Can you work these out from the drawing? Everything is in mm from the part's minimum corner. Round coordinates to 2 decimals unless told otherwise and drop trailing zeros. Write each loop counter-clockwise with the first axis right and the second up, starting at its lowest first coordinate (ties: lowest second). Pieces come first, ordered by that corner, then holes. Notation, with made-up numbers: (-30.75, 8.25) -> (22.25, 8.25) arc R8 ccw to (22.25, 14.25) -> close; hole circle Ø7 at (11, -21). An arc over 180 degrees is marked (long way). Write item = value, one per line. Start each with the question number.
1) Imagine slicing it at B-B, the plane z = 2.5. Please give me the cut outline in (x, y).
2) If I drill on line 1 (Y direction, x = 0.45, z = 5.25), over which ranges is the centre line in solid material (lowest first)?
3) Imagine slicing it at A-A, the plane x = 0.25. Please give me the cut outline in (y, z).
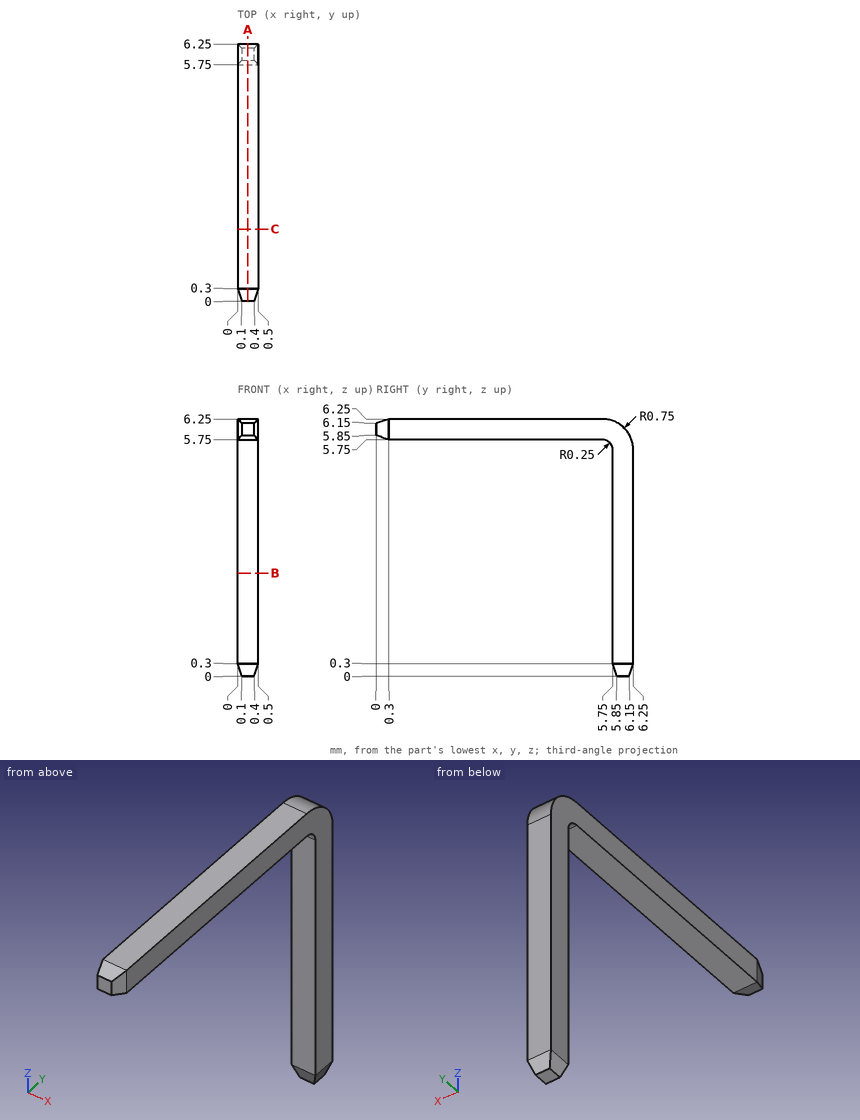
Reported:
q1.outline = (0, 5.75) -> (0.5, 5.75) -> (0.5, 6.25) -> (0, 6.25) -> close
q2.line_1 = 5.75 to 6.25
q3.outline = (0, 5.85) -> (0.3, 5.75) -> (5.5, 5.75) arc R0.25 cw to (5.75, 5.5) -> (5.75, 0.3) -> (5.85, 0) -> (6.15, 0) -> (6.25, 0.3) -> (6.25, 5.5) arc R0.75 ccw to (5.5, 6.25) -> (0.3, 6.25) -> (0, 6.15) -> close
